The model under review builds one solid part; all positions refer to its coordinate system, in mm. A direction names the side the tool comes from. Coordinates: 2 decimals unless noted, no trailing zeros. Order: outer loops, then holes, each group sorted by start corner. A loop starts at its lowest first (then second) coordinate and runs counter-clockwise, first axis right, second up. Notation, with made-up numbers: M 28,17.25 L 76,17.25 A19 cw 76,28.25 Z; hole C 50,33 d10. An arc over 180 degrees is marked long. Answer in a Markdown table with one row per item.
Autodesk Inventor part; units mm, degrees
ref_plane "YZ Plane" through (0, 0, 0) normal (1, 0, 0) x (0, 1, 0)
ref_plane "XZ Plane" through (0, 0, 0) normal (0, 1, 0) x (-1, 0, 0)
ref_plane "XY Plane" through (0, 0, 0) normal (0, 0, 1) x (1, 0, 0)
sketch "Sketch1" plane through (0, 0, 0) normal (0, 1, 0) x (-1, 0, 0)
  line L0 (7.8024, -7.4673) -> (-12.3976, -7.4673)
  line L1 (-12.3976, -7.4673) -> (-12.3976, 14.7327)
  line L2 (-12.3976, 14.7327) -> (7.8024, 14.7327)
  line L3 (7.8024, 14.7327) -> (7.8024, -7.4673)
  line L4 (-12.3976, 0.0327) -> (7.8024, 0.0327)
  line L5 (-12.3976, -3.7208) -> (4.0489, -3.7208)
  line L6 (7.8024, 0.0327) -> (4.0489, -3.7208)
  point P0 (0, 0)
  dimension "d0" = 20.2
  dimension "d1" = 22.2
  dimension "d2" = 14.7
  dimension "d3" = 7.5
  dimension "d4" = 3.7465
  dimension "d5" = 45
extrude "Extrusion1" add sketch "Sketch1" along normal blind 8.5 contours L4 L1 L2 L3 | L6 L5 L1 L4
chamfer "Chamfer1" distance 0.508 angle 45 1 edges at (12.3976, 8.5, 5.506)
chamfer "Chamfer2" distance 0.508 angle 45 1 edges at (3.9204, 8.5, -3.7208)
chamfer "Chamfer3" distance 0.508 angle 45 1 edges at (-7.8024, 8.5, 7.3827)
chamfer "Chamfer4" distance 0.508 angle 45 1 edges at (-5.9256, 8.5, -1.844)
chamfer "Chamfer5" distance 0.508 angle 45 1 edges at (2.2976, 8.5, 14.7327)
chamfer "Chamfer6" distance 0.508 angle 45 5 edges at (-5.9256, 0, -1.844) (-7.8024, 0, 7.3827) (2.2976, 0, 14.7327) (12.3976, 0, 5.506) (4.1744, 0, -3.7208)
sketch "Sketch2" plane through (-7.8024, 7.992, 0.0327) normal (-1, 0, 0) x (0, 0, 1)
  line L0 (0, 0) -> (14.7, 0)
  line L1 (0, -7.484) -> (0.635, -7.484)
  line L2 (0.635, -7.484) -> (0.635, 0)
  line L3 (0.635, 0) -> (0, 0)
  line L4 (0, 0) -> (0, -7.484)
  point P0 (-0.0327, -7.992)
  point P1 (14.7, 0)
  point P2 (1.5266, 1.0795)
  point P3 (13.6205, 0)
  dimension "d26" = 0.635
extrude "Extrusion2" add sketch "Sketch2" along normal blind 1.65 and the other way blind 21.85
chamfer "Chamfer7" distance 0.508 angle 45 1 edges at (12.3976, 4.25, -3.7208)
sketch "Sketch4" plane through (-4.0489, 0.508, -3.7208) normal (0, 0, -1) x (-1, 0, 0)
  line L0 (-15.9385, 0) -> (-15.9385, 7.484)
  line L1 (0, 0) -> (-15.9385, 0)
  line L2 (0, 0) -> (0, 7.484)
  line L3 (-15.9385, 7.484) -> (0, 7.484)
  line L4 (0, 0) -> (-15.9385, 0)
  circle A0 centre (-12.1965, 3.742) radius 3.742
  point P0 (-4.0489, -0.508)
extrude "Extrusion3" add sketch "Sketch4" along normal blind 3.75 contours A0
chamfer "Chamfer8" distance 0.508 angle 45 1 edges at (11.8896, 4.25, -7.4708)
sketch "Sketch5" plane through (8.1476, 4.25, -7.4708) normal (0, 0, -1) x (-1, 0, 0)
  circle A0 centre (0, 0) radius 3.234
  circle A1 centre (0, 0) radius 1.905
  point P0 (8.1476, -4.25)
  dimension "d39" = 3.81
extrude "Extrusion4" add sketch "Sketch5" along normal blind 3.8382 contours A1
sketch "Sketch6" plane through (-4.0489, 0.508, -3.7208) normal (0, 0, -1) x (-1, 0, 0)
  circle A0 centre (-12.1965, 3.742) radius 1.905
  point P0 (-4.0489, -0.508)
sketch "Sketch7" plane through (-4.0489, 0.508, -3.7208) normal (0, 0, -1) x (-1, 0, 0)
  arc A0 (-12.1965, 0) -> (-12.1965, 7.484) centre (-12.1965, 3.742) ccw
  line L0 (0, 0) -> (-12.1965, 0)
  line L1 (0, 0) -> (0, 7.484)
  line L2 (-12.1965, 7.484) -> (0, 7.484)
  circle A1 centre (-12.1965, 3.742) radius 1.905
  circle A2 centre (-12.1965, 3.742) radius 1.905
  circle A3 centre (-12.1965, 3.742) radius 3.234
  circle A4 centre (-12.1965, 3.742) radius 3.234
  arc A5 (-12.1965, 7.484) -> (-15.9385, 3.742) centre (-12.1965, 3.742) ccw
  line L3 (-15.9385, 7.484) -> (-12.1965, 7.484)
  line L4 (-15.9385, 3.742) -> (-15.9385, 7.484)
  line L5 (-15.9385, 3.742) -> (-15.9385, 7.484)
  line L6 (-16.4465, 7.484) -> (-16.4465, 0)
  arc A6 (-15.9385, 3.742) -> (-12.1965, 0) centre (-12.1965, 3.742) ccw
  line L7 (-15.9385, 0) -> (-15.9385, 3.742)
  line L8 (-12.1965, 0) -> (-15.9385, 0)
  line L9 (-16.4465, 7.484) -> (-16.4465, 0)
  line L10 (-18.0965, 7.484) -> (-16.4465, 7.484)
  line L11 (-18.0965, 0) -> (-18.0965, 7.484)
  line L12 (-16.4465, 0) -> (-18.0965, 0)
  point P0 (-4.0489, -0.508)
  dimension "d42" = 5.9
properties part number "HD1440A_Servo"
(1) To check wall thickness, follow line 1 (Z direction, x = 4.25, y = 4.75); line 2 (X direction, y = 1.5, z = 3.25); line 3 (Z direction, x = -8.25, y = 4.5). State the ranges of each line that lie inside material, in increasing order. Write a range as [from, to].
Report:
| item | result |
|---|---|
| line 1 | [-3.72, 14.73] |
| line 2 | [-7.8, 12.4] |
| line 3 | [0.03, 0.67] |
(2) Machinability: for faces 1 (the cylindrical face through (11.117, 6.527, -5.319)), 2 (the flat face through (11, 1, -3.721)), 3 (the flat face through (12.398, 4, -2)), 4 (the flat face through (-7.802, 4, 8)), which of the approach directions +Z, -Z, +X, -X, +Y, -Y give a long, thin tool a straight path to every point of the face, cutting with its end or side? Answer none if there is none.
Report:
| item | result |
|---|---|
| face 1 | -Z |
| face 2 | -Z, +X, -Y |
| face 3 | -Z, +X, +Y, -Y |
| face 4 | +Z, -X, +Y, -Y |
(3) Take a section at C-C (z = -9). Write out the cut boundary in (x, y) (3 decimals).
Report:
| item | result |
|---|---|
| outline | C 8.148,4.25 d3.81 |
(4) Insertion check: P1, Ø3, axis at y = 2.5, z = 8, coming from the -X side; P2, Ø0.7, axis at x = -9, z = 0.5, coming from the -Y side; P3, Ø1.3, axis at x = 13.5, y = 4, coming from the -Z side. Each pin has a flat end and moves straight along its axis. Give the tip position at first contact, or say it passes through.
Report:
| item | result |
|---|---|
| P1 | x = -7.8 |
| P2 | y = 0.51 |
| P3 | z = 0.03 |
(5) Take a section at A-A (x = 4). Write out the cut boundary in (y, z), then the cut area to 3 significant figures.
Report:
| item | result |
|---|---|
| outline | M 0,-3.21 L 0.51,-3.72 L 7.99,-3.72 L 8.5,-3.21 L 8.5,14.22 L 7.99,14.73 L 0.51,14.73 L 0,14.22 Z |
| area | 156 mm^2 |
(6) Take a section at B-B (z = 8.75). Write out the cut boundary in (x, y).
Report:
| item | result |
|---|---|
| outline | M -7.8,0.51 L -7.29,0 L 11.89,0 L 12.4,0.51 L 12.4,7.99 L 11.89,8.5 L -7.29,8.5 L -7.8,7.99 Z |
